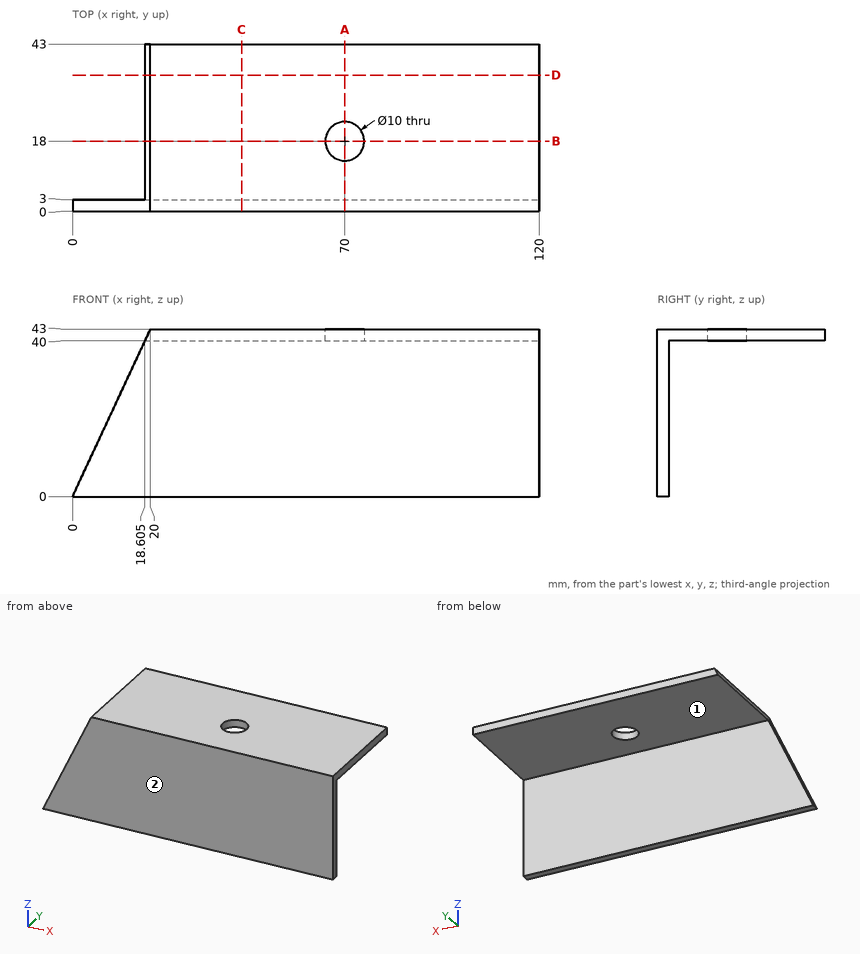
Can you work these out from the drawing? Everything is in mm from the part's minimum corner. A direction names the side the tool comes from. Round coordinates to 2 decimals unless told otherwise and drop trailing zeros. Loops run counter-clockwise (first coordinate to the right, second up) from the corner with the lowest first, then second, coordinate; pieces in that order, holes last. Notation, with made-up numbers: (67.5, 80) - (122.5, 80) arc R11 cw to (122.5, 89) - close; hole circle Ø9 at (64, 5.5). An arc over 180 degrees is marked (long way). One line per question, with ' | ' between items. Start each with the question number.
Q1. I want a section at A-A (x = 70). Write out the boundary of the cut face in (y, z), then the cut area to 3 significant figures.
Q2. I want a section at C-C (x = 43.5). Write out the boundary of the cut face in (y, z).
Q3. For the marked faces 1 and 2, which set-ups out of +Z, -Z, +X, -X, +Y, -Y let a thin tool reach every point of the face, with its end or its side?
Q4. I want a section at B-B (y = 18). Write out the boundary of the cut face in (x, z) (1 decimal), then the cut area to 3 significant figures.
Q5. Will these pins go through, and if not, where does the flat tip stop? pin 1 (1.5 mm diameter, centred on x = 31, z = 28.5, fed in from +Y); pin 2 (13 mm diameter, centred on x = 70, y = 18, fed in from -Z).
Q6. Please list where these lines run through material, in increasing order: line 1 (Y direction, x = 70, z = 41); line 2 (Y direction, x = 26, z = 25.5); line 3 (Z direction, x = 95.5, y = 17). Write a range as [from, to].
Q7. I want a section at D-D (y = 35). Write out the boundary of the cut face in (x, z) (1 decimal).
Response values:
1) outline: (0, 0) - (3, 0) - (3, 40) - (13, 40) - (13, 43) - (0, 43) - close; (23, 40) - (43, 40) - (43, 43) - (23, 43) - close | area: 219 mm²
2) outline: (0, 0) - (3, 0) - (3, 40) - (43, 40) - (43, 43) - (0, 43) - close
3) face 1: -Z, +X, -X, +Y | face 2: +Z, -Z, +X, -X, -Y
4) outline: (18.6, 40) - (65, 40) - (65, 43) - (20, 43) - close; (75, 40) - (120, 40) - (120, 43) - (75, 43) - close | area: 272 mm²
5) pin 1: stops at y = 3 | pin 2: stops at z = 40
6) line 1: y = [0, 13], [23, 43] | line 2: y = [0, 3] | line 3: z = [40, 43]
7) outline: (18.6, 40) - (120, 40) - (120, 43) - (20, 43) - close
